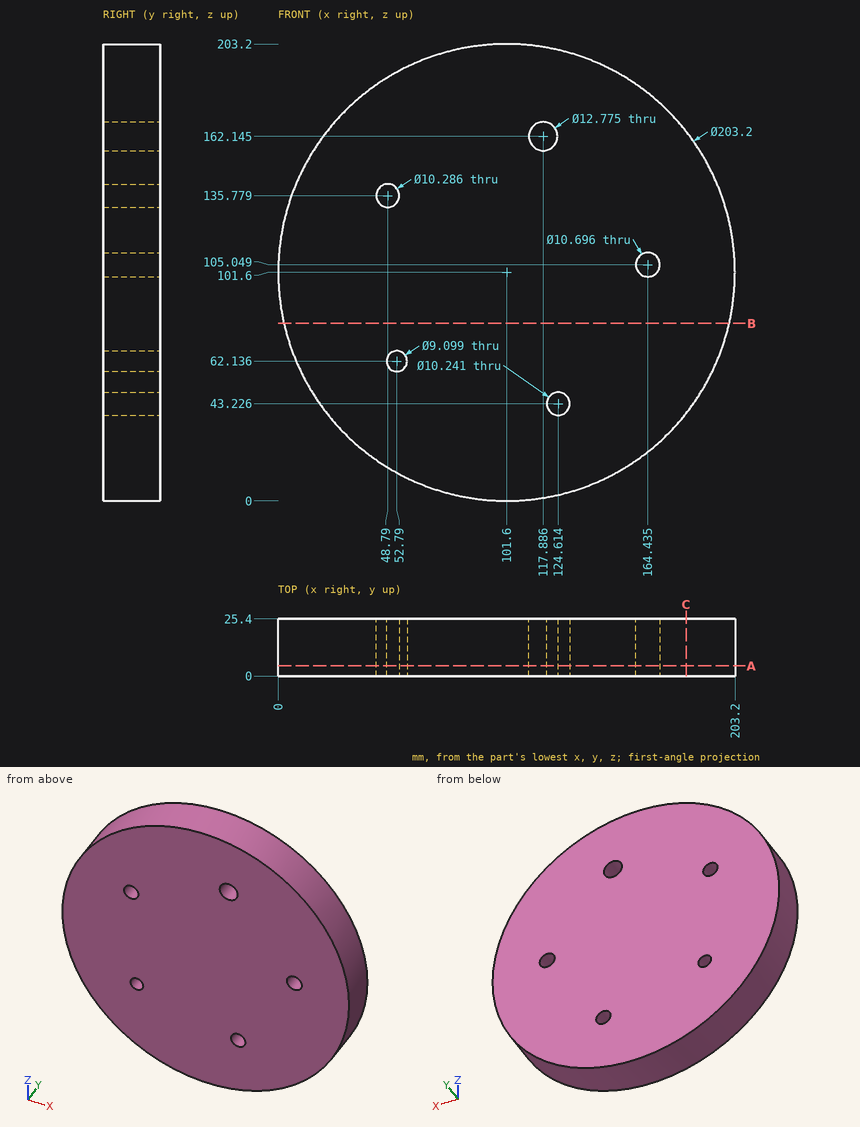
The figure shows three views and two pictorial views of one solid part (mm, origin at its lowest corner). Answer the questions. Give positions to 0.01 mm unless a question says otherwise; leave off trailing zeros. Order: outer loops, then holes, each group sorted by start corner. A loop starts at its lowest first (then second) coordinate and runs counter-clockwise, first axis right, second up. Notation, with made-up numbers: (-6.5, 4) -> (23.5, 4) arc R6 ccw to (23.5, 9) -> close; hole circle Ø10 at (37.25, 54.5). An arc over 180 degrees is marked (long way). One line per item, written item: value.
1) Find section C-C, the plane x = 181.5. Determine the outline of the cut face in (y, z), plus the area to 3 significant figures.
Reported:
outline: (0, 38.84) -> (25.4, 38.84) -> (25.4, 164.36) -> (0, 164.36) -> close
area: 3,190 mm^2
2) Find section A-A, the plane y = 4.5. Count the separate pieces of the cut face and the enclosed holes in it, plus the area to 3 significant figures.
Reported:
separate pieces: 1
enclosed holes: 5
area: 32,000 mm^2
3) Find the intervals of material crossed by line 1 (Z direction, x = 122, y = 7) (1 decimal); line 2 (Z direction, x = 55.5, y = 10.25); line 3 (Z direction, x = 162.5, y = 5.25) (1 decimal), in increasing order.
Reported:
line 1: z = 2.1 to 38.8, 47.6 to 157.3, 167 to 201.1
line 2: z = 11.06 to 58.48, 65.79 to 192.14
line 3: z = 20.3 to 100.1, 110 to 182.9
4) Find section B-B, the plane z = 79. Determine the outline of the cut face in (x, y) (1 decimal), plus the area to 3 significant figures.
Reported:
outline: (2.5, 0) -> (200.7, 0) -> (200.7, 25.4) -> (2.5, 25.4) -> close
area: 5,030 mm^2
5) Flat-ended cylindrical pins translate along their axes: P1, Ø5, axis at y = 7, z = 109, coming from the +X side; P2, Ø1, axis at x = 39.5, y = 4.5, coming from the +Z side (1 decimal); P3, Ø5, axis at x = 28, y = 6, coming from the -Z side (1 decimal). Find the tip coordinate at first contact, or state that the pin passes through.
Reported:
P1: stops at x = 203.08
P2: stops at z = 182.4
P3: stops at z = 29
